Source: CAD feature listing. Evaluate the final solid. Frame: model axes, mm. A direction names the side the tool comes from. Coordinates: 2 decimals unless noted, no trailing zeros. Order: outer loops, then holes, each group sorted by start corner. A loop starts at its lowest first (then second) coordinate and runs counter-clockwise, first axis right, second up. Notation, with made-up numbers: (70.5, 16.25) -> (118.5, 16.25) arc R21 ccw to (118.5, 26.25) -> close; hole circle Ø3 at (26, 65). An arc over 180 degrees is marked (long way). Put each result on its own line as item: value.
from build123d import *

# Parameters (mm, degrees)
CUT_EXTRUDE1_DEPTH = 31.4452


with BuildPart() as part:
    # Sketch1 → Revolve1 (revolve)
    with BuildSketch(Plane.XY):
        with BuildLine():
            Line((0, 0), (0, 4.79425))
            Line((0, 4.79425), (0.762, 5.55625))
            Line((0.762, 5.55625), (18.912356192, 5.55625))
            Line((18.912356192, 5.55625), (19.651103096, 4.817503096))
            ThreePointArc((19.651103096, 4.817503096), (19.923034747, 4.635804176), (20.2438, 4.572))
            Line((20.2438, 4.572), (21.3868, 4.572))
            ThreePointArc((21.3868, 4.572), (21.979496904, 4.817503096), (22.225, 5.4102))
            Line((22.225, 5.4102), (22.225, 7.8486))
            Line((22.225, 7.8486), (30.1752, 7.8486))
            Line((30.1752, 7.8486), (30.1752, 0))
            Line((30.1752, 0), (0, 0))
        make_face()
    revolve(axis=Axis((30.1752, 0, 0), (-1, 0, 0)))

    # Sketch3 → Revolve2 (revolve)
    with BuildSketch(Plane.XY):
        with BuildLine():
            Line((30.1752, 0), (30.1752, 6.2484))
            ThreePointArc((30.1752, 6.2484), (30.435582072, 5.619782072), (31.0642, 5.3594))
            Line((31.0642, 5.3594), (32.1564, 5.3594))
            ThreePointArc((32.1564, 5.3594), (32.496605571, 5.427071096), (32.785017928, 5.619782072))
            Line((32.785017928, 5.619782072), (33.515235857, 6.35))
            Line((33.515235857, 6.35), (54.81955, 6.35))
            Line((54.81955, 6.35), (55.5752, 5.59435))
            Line((55.5752, 5.59435), (55.5752, 0))
            Line((55.5752, 0), (30.1752, 0))
        make_face()
    revolve(axis=Axis((55.5752, 0, 0), (-1, 0, 0)))

    # Sketch2 → Cut-Extrude1 (cut)
    with BuildSketch(Plane(origin=(0, 0, 0), x_dir=(0, 0, -1), z_dir=(1, 0, 0))):
        Polygon((-21.859138511, -5.857138511), (5.857138511, -21.859138511), (21.859138511, 5.857138511), (-5.857138511, 21.859138511), align=None)
        with BuildLine():
            Line((2.227168484, -8.842431029), (8.771354144, 2.492431029))
            ThreePointArc((8.771354144, 2.492431029), (4.5593, 7.896939247), (-2.227168484, 8.842431029))
            Line((-2.227168484, 8.842431029), (-8.771354144, -2.492431029))
            ThreePointArc((-8.771354144, -2.492431029), (-4.5593, -7.896939247), (2.227168484, -8.842431029))
        make_face(mode=Mode.SUBTRACT)
    extrude(amount=CUT_EXTRUDE1_DEPTH, mode=Mode.SUBTRACT)


solid = part.part
1. First-contact query: pin 1 (8 mm diameter, centred on x = 44.5, z = -1.5, fed in from -Y); pin 2 (8 mm diameter, centred on x = 39, y = 5.5, fed in from -Z); pin 3 (4 mm diameter, centred on x = 12.5, z = 1, fed in from -Y). Flat tips, straight axial feed; report the tip coordinate or a pass-through.
Numbers:
pin 1: stops at y = -6.35
pin 2: stops at z = -6.17
pin 3: stops at y = -5.56
2. Pull-direction query (X, two-part tool) for faces 3 (the cylindrical face through (20.823, -0.991, 4.463)), 4 (the cylindrical face through (9.96, 5.3, -1.67)), 5 (the cylindrical face through (31.618, -5.354, -0.236)), 6 (the flat face through (55.575, 0, 0)); classes: pulls with the +X half, pulls with the -X half, needs draft (parallel to the pull), parting line crosses it, or undercut.
Numbers:
face 3: undercut
face 4: needs draft
face 5: undercut
face 6: pulls with the +X half
3. Ray query, line 1 along Z through (x, y) = (51, 0); line 2 along X through (y, z) = (-4.5, 1.25); line 3 along X through (y, z) = (6.5, -2.75) (3 decimals). Return the intervals inside material, ascending.
Numbers:
line 1: z = -6.35 to 6.35
line 2: x = 0 to 19.85, 21.78 to 55.58
line 3: x = 22.225 to 30.175
4. Set-up query: faces 1 (the flat face through (0, 0, 0)), 2 (the cylindrical face through (44.32, -1.38, 6.2)). Return all of +Z, -Z, +X, -X, +Y, -Y with unobstructed straight access to the full face (end or side cutting, diameter ignored); none if empty.
Numbers:
face 1: +Z, -Z, -X, +Y, -Y
face 2: +X
5. Cut plane C-C on x = 52.5. Output: boundary loops of the cut face in (y, z).
Numbers:
outline: circle Ø12.7 at (0, 0)
